Part model, mm, in its own coordinate system. Face numbers are marked on the shaded views. A direction names the side the tool comes from. Coordinates: 2 decimals unless noted, no trailing zeros. Loops run counter-clockwise (first coordinate to the right, second up) from the corner with the lowest first, then second, coordinate; pieces in that order, holes last. Notation, with made-up numbers: M 54.5,57.5 L 82.5,57.5 A5 ccw 82.5,63.5 Z; hole C 26.5,50 d2. An arc over 180 degrees is marked long. Answer as a JSON object with one key per item and string values. Group by question number.
1. Drop flat-ended pins along their axis: pin 1 Ø12 at (y, z) = (26.5, -11.5) entering from -X; pin 2 Ø1.5 at (y, z) = (21.5, -5) entering from +X; pin 3 Ø4 at (x, y) = (-6, 16) entering from -Z. Give the stop position or say it passes through.
2. Saw through at A-A on x = 0. Write the cut outline in (y, z), then the cut area to 3 significant figures.
3. Drill centre lines: L1, parallel to X at y = -3, z = -18; L2, parallel to X at y = 27.5, z = -5.25; L3, parallel to Y at x = 5.5, z = -15.75. Where is each one in solid material? Low to high.
4. 3-axis set-ups, long thin cutter, end or side, ignore diameter. For the marked faces 1, 2, 3 and 4: which of +Z, -Z, +X, -X, +Y, -Y reach the whole face in a straight line?
5. Saw through at B-B on y = 1. Write the cut outline in (x, z).
6. Saw through at C-C on y = 30. Write the cut outline in (x, z), then the cut area to 3 significant figures.
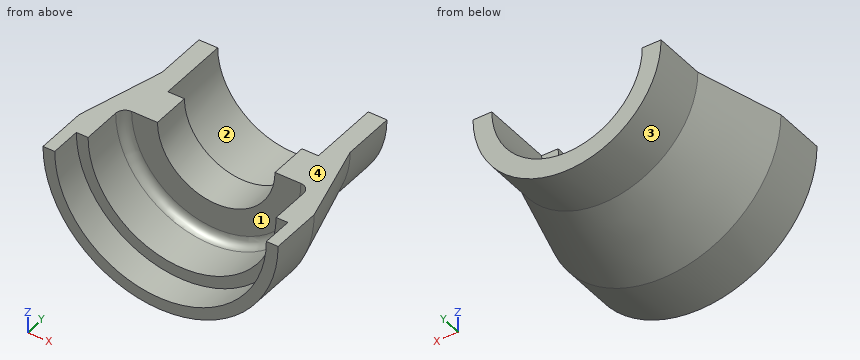
from build123d import *

# Parameters (mm, degrees)
SKETCH3_W          = 71.408394521
SKETCH3_H          = 27.275546844
CUT_EXTRUDE2_DEPTH = 100


with BuildPart() as part:
    # Sketch1 → Revolve1 (revolve)
    with BuildSketch(Plane.XY, mode=Mode.PRIVATE) as revolve1_sk:
        with BuildLine():
            Line((16, 32.849548789), (16, 17.609057399))
            Line((16, 17.609057399), (12.5, 17.609057399))
            Line((12.5, 17.609057399), (12.5, 9.374527929))
            Line((12.5, 9.374527929), (18, 9.374527929))
            ThreePointArc((18, 9.374527929), (19.414213562, 8.788741491), (20, 7.374527929))
            Line((20, 7.374527929), (20, -1.061426296))
            Line((20, -1.061426296), (22.5, -1.061426296))
            Line((22.5, -1.061426296), (22.5, -7.65813411))
            Line((22.5, -7.65813411), (25, -7.65813411))
            Line((25, -7.65813411), (25, 3.380682237))
            Line((25, 3.380682237), (20, 21.59503207))
            Line((20, 21.59503207), (20, 32.849548789))
            Line((20, 32.849548789), (16, 32.849548789))
        make_face()
    revolve(revolve1_sk.sketch.rotate(Axis((0, 89.637369386, 0), (0, -1, 0)), 90), axis=Axis((0, 89.637369386, 0), (0, -1, 0)))  # turned: the seam where the file's is

    # Sketch3 → Cut-Extrude2 (cut, symmetric)
    with BuildSketch(Plane(origin=(0, 0, 0), x_dir=(1, 0, 0), z_dir=(0, 1, 0))):
        with Locations((-0.506442515, -13.637773422)):
            Rectangle(SKETCH3_W, SKETCH3_H)
    extrude(amount=CUT_EXTRUDE2_DEPTH, both=True, mode=Mode.SUBTRACT)


solid = part.part
Outcome:
{
 "1": {"pin 1": "stops at x = -19.23", "pin 2": "stops at x = 19.67", "pin 3": "stops at z = -21.44"},
 "2": {"outline": "M -7.66,-25 L 3.38,-25 L 21.6,-20 L 32.85,-20 L 32.85,-16 L 17.61,-16 L 17.61,-12.5 L 9.37,-12.5 L 9.37,-18 A2 cw 7.37,-20 L -1.06,-20 L -1.06,-22.5 L -7.66,-22.5 Z", "area": "208 mm²"},
 "3": {"L1": "x = -17.35 to -13.5, 13.5 to 17.35", "L2": "x = -19.3 to -15.11, 15.11 to 19.3", "L3": "y = 9.37 to 32.85"},
 "4": {"face 1": "+Z, -Y", "face 2": "+Z, +Y", "face 3": "-Z, +Y", "face 4": "+Z, +X, -X, +Y, -Y"},
 "5": {"outline": "M -25,0 A25 ccw 25,0 L 20,0 A20 cw -20,0 Z"},
 "6": {"outline": "M -20,0 A20 ccw 20,0 L 16,0 A16 cw -16,0 Z", "area": "226 mm²"}
}
